Autodesk Inventor part; units mm, degrees
ref_plane "YZ Plane" through (0, 0, 0) normal (1, 0, 0) x (0, 1, 0)
ref_plane "XZ Plane" through (0, 0, 0) normal (0, 1, 0) x (-1, 0, 0)
ref_plane "XY Plane" through (0, 0, 0) normal (0, 0, 1) x (1, 0, 0)
sketch "Sketch1" plane through (0, 0, 0) normal (0, 0, 1) x (1, 0, 0)
  line L0 (0, 117.6) -> (0, -117.6)
  line L1 (-194.6, 0) -> (194.6, 0)
  line L2 (-89, 84) -> (89, 84)
  line L3 (139, 34) -> (139, -34)
  line L4 (89, -84) -> (-89, -84)
  line L5 (-139, -34) -> (-139, 34)
  circle A0 centre (-95, 0) radius 25
  circle A1 centre (95, 0) radius 25
  circle A2 centre (0, 0) radius 45
  line L6 (-89, 84) -> (-139, 34)
  line L7 (89, 84) -> (139, 34)
  line L8 (139, -34) -> (89, -84)
  line L9 (-89, -84) -> (-139, -34)
  point P0 (-139, 84)
  point P1 (139, 84)
  point P2 (-139, -84)
  point P3 (139, -84)
  dimension "d0" = 278
  dimension "d1" = 168
  dimension "d8" = 50
  dimension "d9" = 190
  dimension "d10" = 95
  dimension "d11" = 90
  dimension "d12" = 50
  dimension "d13" = 50
  dimension "d14" = 50
  dimension "d15" = 50
  dimension "d16" = 50
  dimension "d17" = 50
  dimension "d18" = 50
  dimension "d19" = 50
extrude "Extrusion2" add sketch "Sketch1" against normal blind 10 contours L2 L7 L3 L1 A1 A2 L0 | L0 A2 L1 A0 L5 L6 L2 | L1 A1 L3 L8 L4 L0 A2 | A2 L0 L4 L9 L5 L1 A0
properties part number "SlipersLåda 211018004"
Input: part model. Units: mm. Frame: model coordinates. Coordinates: 2 decimals unless noted, no trailing zeros. Write each loop counter-clockwise with the first axis right and the second up, starting at its lowest first coordinate (ties: lowest second). Pieces come first, ordered by that corner, then holes. Notation, with made-up numbers: M 68.25,57 L 81.25,57 A15 ccw 81.25,71 Z; hole C 22.5,10.25 d2. An arc over 180 degrees is marked long. Answer as a JSON object with one key per item and string values. Group by question number.
(1) Ray query, line 1 along X through (y, z) = (0, -2.5); line 2 along Y through (x, z) = (0, -8); line 3 along Y through (x, z) = (-16, -8). Return the intervals inside material, ascending. Write a range as [from, to].
(2) Mould query, pull axis X, two halves, no side actions, for faces 1 (the face through (20.765, -39.923, -4.93)), 2 (the face through (114, -59, -5)), 3 (the face through (-33, 39, -10)). Classes: pulls with the +X half, pulls with the -X half, needs draft (parallel to the pull), parting line crosses it, or undercut.
(3) Section B-B on y = 0. Output: boundary loops of the cut face in (x, z), plus the area to 3 significant figures.
(4) Section C-C on z = -6.75. Output: boundary loops of the cut face in (x, y), plus the area to 3 significant figures.
(5) Section D-D on x = -95. Output: boundary loops of the cut face in (y, z).
(6) Contact query for a flat-ended pin moving along its axis: P1, Ø1, axis at y = 57, z = -9, coming from the +X side. Output: stop coordinate, or through.
(7) Section A-A on x = 0. Output: boundary loops of the cut face in (y, z).
Result set:
{
 "1": {"line 1": "x = [-139, -120], [-70, -45], [45, 70], [120, 139]", "line 2": "y = [-84, -45], [45, 84]", "line 3": "y = [-84, -42.06], [42.06, 84]"},
 "2": {"face 1": "undercut", "face 2": "pulls with the +X half", "face 3": "needs draft"},
 "3": {"outline": "M -139,-10 L -120,-10 L -120,0 L -139,0 Z; M -70,-10 L -45,-10 L -45,0 L -70,0 Z; M 45,-10 L 70,-10 L 70,0 L 45,0 Z; M 120,-10 L 139,-10 L 139,0 L 120,0 Z", "area": "880 mm2"},
 "4": {"outline": "M -139,-34 L -89,-84 L 89,-84 L 139,-34 L 139,34 L 89,84 L -89,84 L -139,34 Z; hole C -95,0 d50; hole C 0,0 d90; hole C 95,0 d50", "area": "31,400 mm2"},
 "5": {"outline": "M -78,-10 L -25,-10 L -25,0 L -78,0 Z; M 25,-10 L 78,-10 L 78,0 L 25,0 Z"},
 "6": {"P1": "stops at x = 116.5"},
 "7": {"outline": "M -84,-10 L -45,-10 L -45,0 L -84,0 Z; M 45,-10 L 84,-10 L 84,0 L 45,0 Z"}
}
